Work out the finished part from the listing and answer in its coordinate system (mm). A direction names the side the tool comes from. Give positions to 0.01 mm unless a question says otherwise; leave off trailing zeros. Order: outer loops, then holes, each group sorted by start corner. A loop starts at its lowest first (then second) coordinate and runs counter-clockwise, first axis right, second up. Notation, with made-up numbers: (-23, 86.25) - (-3, 86.25) arc R20 ccw to (-3, 107.25) - close; hole circle Ø2 at (-20.5, 24). An arc over 180 degrees is marked (long way). Write each question's results on one line, items separated by ' | '.
Autodesk Inventor part; units mm, degrees
ref_plane "YZ Plane" through (0, 0, 0) normal (1, 0, 0) x (0, 1, 0)
ref_plane "XZ Plane" through (0, 0, 0) normal (0, 1, 0) x (-1, 0, 0)
ref_plane "XY Plane" through (0, 0, 0) normal (0, 0, 1) x (1, 0, 0)
sketch "スケッチ1" plane through (0, 0, 0) normal (0, 0, 1) x (1, 0, 0)
  line L0 (0, 0) -> (0, -12)
  line L1 (0, -12) -> (-2, -40)
  line L2 (-2, -40) -> (-28, -40)
  line L3 (-28, -40) -> (-30, -12)
  line L4 (-30, -12) -> (-30, 0)
  line L5 (-30, 0) -> (0, 0)
  circle A0 centre (-25, -5) radius 1.75
  circle A1 centre (-5, -5) radius 1.75
  dimension "d0" = 12
  dimension "d1" = 30
  dimension "d2" = 40
  dimension "d3" = 2
  dimension "d4" = 26
  dimension "d12" = 3.5
  dimension "d13" = 3.5
  dimension "d14" = 5
  dimension "d15" = 5
  dimension "d16" = 5
extrude "押し出し1" add sketch "スケッチ1" along normal blind 20
sketch "スケッチ2" plane through (0, -12, 0) normal (1, 0, 0) x (0, 0, -1)
  line L0 (0, 12) -> (-20, 12)
  line L1 (-3, 12) -> (-13.5, 12)
  line L2 (-13.5, 12) -> (-13.5, 1.5)
  line L3 (-13.5, 1.5) -> (-3, 1.5)
  line L4 (-3, 1.5) -> (-3, 12)
  line L5 (0, 12) -> (0, 0)
  line L6 (0, -28) -> (0, 0)
  line L7 (0, 0) -> (-12, -28)
  line L8 (0, -28) -> (-20, -28)
  circle A0 centre (-16, -23) radius 1.75
  line L9 (-20, -28) -> (-20, 0)
  dimension "d7" = 10.5
  dimension "d8" = 10.5
  dimension "d9" = 3
  dimension "d22" = 12
  dimension "d34" = 3.5
  dimension "d35" = 4
  dimension "d36" = 5
extrude "押し出し2" cut sketch "スケッチ2" against normal through all
sketch "スケッチ3" plane through (0, 0, 0) normal (0, 0, -1) x (-1, 0, 0)
  line L0 (4, -40) -> (26, -40)
  line L1 (26, -40) -> (26, -16.5)
  line L2 (26, -16.5) -> (4, -16.5)
  line L3 (4, -16.5) -> (4, -40)
  line L4 (28, -40) -> (2, -40)
  point P0 (0, 0)
  dimension "d17" = 23.5
  dimension "d18" = 2
  dimension "d19" = 2
extrude "押し出し3" cut sketch "スケッチ3" against normal blind 12
sketch "スケッチ4" plane through (0, 0, 20) normal (0, 0, 1) x (1, 0, 0)
  line L0 (-22.5, -30) -> (-7.5, -30)
  line L1 (-7.5, -30) -> (-7.5, -20)
  line L2 (-7.5, -20) -> (-22.5, -20)
  line L3 (-22.5, -20) -> (-22.5, -30)
  line L4 (0, 0) -> (-30, 0)
  line L5 (0, -12) -> (0, 0)
  dimension "d23" = 15
  dimension "d24" = 20
  dimension "d25" = 7.5
  dimension "d26" = 10
hole "穴1" at (-22.5, -20, 20) at (-22.5, -30, 20) at (-7.5, -30, 20) at (-7.5, -20, 20) direction (0, 0, -1) diameter 3.2 end through all
fillet "フィレット1" radius 2 7 edges at (-26, -16.5, 6.9643) (-4, -16.5, 6.9643) (-15, -40, 12) (-3, -40, 12) (-27, -40, 12) (0, -12, 10) (-30, -12, 10)
fillet "フィレット2" radius 2 4 edges at (0, 0, 16.75) (0, 0, 1.5) (-30, 0, 1.5) (-30, 0, 16.75)
properties part number "ma_3d1"
1. A tool of negligible diameter and unlimited length cuts with its end or side. For faces 5 (the face through (-14.85, -39.43, 12.6)), 6 (the face through (-14.79, -16.277, 1.833)), 7 (the face through (-15, -10.5, 8)), from which of +Z, -Z, +X, -X, +Y, -Y can it reach the whole face along a straight path? Write none if from no direction.
Answer list:
face 5: -Z, -Y | face 6: -Z, +X, -X, -Y | face 7: +X, -X, +Y
2. A cutting plane is placed at D-D, the plane z = 16. Write down the section's boundary in (x, y), then the cut area to 3 significant figures.
Answer list:
outline: (-30, -11.93) arc R2 ccw to (-29.99, -12.07) - (-28.48, -33.25) - (-1.52, -33.25) - (-0.01, -12.07) arc R2 ccw to (0, -11.93) - (0, -2) arc R2 ccw to (-2, 0) - (-28, 0) arc R2 ccw to (-30, -2) - close; (-28.23, -36.75) - (-28, -40) - (-2, -40) - (-1.77, -36.75) - close; hole circle Ø3.5 at (-25, -5); hole circle Ø3.2 at (-22.5, -30); hole circle Ø3.2 at (-22.5, -20); hole circle Ø3.2 at (-7.5, -30); hole circle Ø3.2 at (-7.5, -20); hole circle Ø3.5 at (-5, -5) | area: 997 mm^2
3. Determine the mould class of faces 1 (the face through (-14.811, -34.474, 14.331)), 2 (the face through (-15, -5, 3)), 3 (the face through (-4, -24, 8)), 4 (the face through (-15, -27, 12)) for opening direction Z: +Z half, -Z half, draft (parallel to the pull), parting line (faces both ways), or undercut.
Answer list:
face 1: undercut | face 2: undercut | face 3: draft | face 4: -Z half
4. A cutting plane is placed at B-B, the plane y = -9.5. Write down the section's boundary in (x, z).
Answer list:
outline: (-30, 0) - (0, 0) - (0, 3) - (-30, 3) - close; (-30, 13.5) - (0, 13.5) - (0, 20) - (-30, 20) - close
5. A cutting plane is placed at C-C, the plane x = -10.75. Write down the section's boundary in (y, z).
Answer list:
outline: (-40, 14) arc R2 ccw to (-38, 12) - (-16.5, 12) - (-16.5, 1.93) - (-12, 0) - (0, 0) - (0, 3) - (-10.5, 3) - (-10.5, 13.5) - (0, 13.5) - (0, 20) - (-40, 20) - close; hole circle Ø3.5 at (-35, 16)
6. Given P1, Ø3, axis at y = -8.5, z = 10, coming from the -X side; P2, Ø1, axis at y = -34.5, z = 14, coming from the -X side; P3, Ø6, axis at x = -17, z = 6, coming from the -Y side; P4, Ø6, axis at y = -19.5, z = 13.5, coming from the -X side, each flat-ended and moving along its own axis, determine where each tip first touches the part or whether it passes through.
Answer list:
P1: through | P2: x = -28.43 | P3: y = -16.5 | P4: x = -29.68
7. Straight lines are drawn through the part: line 1 (Y direction, x = -5, z = 18.5); line 2 (Y direction, x = -7.5, z = 14.5); line 3 (Z direction, x = -22.25, y = -3.5). For each, find the intervals that lie inside material, in ascending order. Write a range as [from, to].
Answer list:
line 1: [-40, -6.75], [-3.25, 0] | line 2: [-40, -35.9], [-34.1, -31.6], [-28.4, -21.6], [-18.4, 0] | line 3: [0, 3], [13.5, 20]
8. A cutting plane is placed at A-A, the plane x = -7.5. Write down the section's boundary in (y, z).
Answer list:
outline: (-40, 14) arc R2 ccw to (-38, 12) - (-31.6, 12) - (-31.6, 20) - (-40, 20) - close; (-28.4, 12) - (-21.6, 12) - (-21.6, 20) - (-28.4, 20) - close; (-18.4, 12) - (-16.5, 12) - (-16.5, 1.93) - (-12, 0) - (0, 0) - (0, 3) - (-10.5, 3) - (-10.5, 13.5) - (0, 13.5) - (0, 20) - (-18.4, 20) - close; hole circle Ø3.5 at (-35, 16)
